Geometry: final body of the model. Coordinates: model frame, mm. Round coordinates to 2 decimals unless told otherwise and drop trailing zeros. Loops run counter-clockwise (first coordinate to the right, second up) from the corner with the lowest first, then second, coordinate; pieces in that order, holes last. Notation, with made-up numbers: (3, 82.25) - (54, 82.25) arc R12 cw to (54, 95.25) - close; hole circle Ø11 at (-30, -2.75). An arc over 180 degrees is marked (long way). Return JSON: item names as keys, results as strings. Group by question number.
1. Section D-D on x = 3. Return loops of the section in (y, z), and give its area (3 significant figures).
2. Draft query along Y for faces 1 (the face through (-1, -63.5, 2)), 2 (the face through (7, 9, 1.27)), 3 (the face through (63.5, -1, 2)). Return one class per face: +Y half, -Y half, draft (parallel to the pull), parting line (faces both ways), or undercut.
3. First-contact query: pin 1 Ø3 at (x, y) = (8, -14.5) entering from +Z. Flat tip, straight axial feed; report the tip coordinate or a pass-through.
4. Section C-C on z = 2.75. Return loops of the section in (x, y), and give its area (3 significant figures).
5. Material intervals for probe 1 along Y at (x, z) = (26.5, 1.55); probe 2 along X at (y, z) = (-8.5, 3); probe 3 along X at (y, z) = (48, 3.2), sorted ascending.
6. Section A-A on y = -27. Return loops of the section in (x, z).
7. Section B-B on x = 44. Return loops of the section in (y, z), and give its area (3 significant figures).
from build123d import *

# Parameters (mm, degrees)
F0_W     = 127
F0_H     = 127
F1_DEPTH = 3.81
F3_DEPTH = 2.54
F5_DEPTH = 2.54


with BuildPart() as f1:
    # F0 (on Top) → F1 (new body)
    with BuildSketch(Plane.XY):
        Rectangle(F0_W, F0_H)
    extrude(amount=F1_DEPTH)

    # F2 (on face) → F3 (cut)
    with BuildSketch(Plane.XY.offset(3.81)):
        Polygon((-53.991713, 52.186977), (-53.991713, -63.5), (-44.085711, -63.5), (-44.085711, 42.280976), (-30.810868, 42.280976), (-30.810868, -41.3385), (30.810867, -41.3385), (30.810867, -7.389393), (9.906001, -7.389393), (9.906001, 6.186236), (47.354292, 6.186236), (47.354292, 33.237237), (37.448291, 33.237237), (37.448291, 16.092237), (0, 16.092237), (0, -17.295394), (20.904865, -17.295394), (20.904865, -31.432498), (-20.904867, -31.432498), (-20.904867, 52.186977), align=None)
    extrude(amount=-F3_DEPTH, mode=Mode.SUBTRACT)

    # F4 (on face) → F5 (cut)
    with BuildSketch(Plane.XY.offset(3.81)):
        Polygon((37.448291, 33.237237), (47.354292, 33.237237), (47.354292, 54.593291), (11.279603, 54.593291), (11.279603, 33.237237), align=None)
    extrude(amount=-F5_DEPTH, mode=Mode.SUBTRACT)


solid = f1.part
Taken from the geometry:
{
 "1": {"outline": "(-63.5, 0) - (63.5, 0) - (63.5, 3.81) - (16.09, 3.81) - (16.09, 1.27) - (-17.3, 1.27) - (-17.3, 3.81) - (-31.43, 3.81) - (-31.43, 1.27) - (-41.34, 1.27) - (-41.34, 3.81) - (-63.5, 3.81) - close", "area": "374 mm2"},
 "2": {"face 1": "-Y half", "face 2": "undercut", "face 3": "draft"},
 "3": {"pin 1": "z = 1.27"},
 "4": {"outline": "(-63.5, -63.5) - (-53.99, -63.5) - (-53.99, 52.19) - (-20.9, 52.19) - (-20.9, -31.43) - (20.9, -31.43) - (20.9, -17.3) - (0, -17.3) - (0, 16.09) - (37.45, 16.09) - (37.45, 33.24) - (11.28, 33.24) - (11.28, 54.59) - (47.35, 54.59) - (47.35, 6.19) - (9.91, 6.19) - (9.91, -7.39) - (30.81, -7.39) - (30.81, -41.34) - (-30.81, -41.34) - (-30.81, 42.28) - (-44.09, 42.28) - (-44.09, -63.5) - (63.5, -63.5) - (63.5, 63.5) - (-63.5, 63.5) - close", "area": "11,400 mm2"},
 "5": {"probe 1": "-63.5 to -41.34, -7.39 to 6.19, 16.09 to 33.24, 54.59 to 63.5", "probe 2": "-63.5 to -53.99, -44.09 to -30.81, -20.9 to 0, 30.81 to 63.5", "probe 3": "-63.5 to -53.99, -20.9 to 11.28, 47.35 to 63.5"},
 "6": {"outline": "(-63.5, 0) - (63.5, 0) - (63.5, 3.81) - (30.81, 3.81) - (30.81, 1.27) - (20.9, 1.27) - (20.9, 3.81) - (-20.9, 3.81) - (-20.9, 1.27) - (-30.81, 1.27) - (-30.81, 3.81) - (-44.09, 3.81) - (-44.09, 1.27) - (-53.99, 1.27) - (-53.99, 3.81) - (-63.5, 3.81) - close"},
 "7": {"outline": "(-63.5, 0) - (63.5, 0) - (63.5, 3.81) - (54.59, 3.81) - (54.59, 1.27) - (6.19, 1.27) - (6.19, 3.81) - (-63.5, 3.81) - close", "area": "361 mm2"}
}
